from build123d import *

# Parameters (mm, degrees)
SKETCH1_R           = 1.2
BOSS_EXTRUDE1_DEPTH = 1.778
CUT_EXTRUDE1_REACH  = 20.691


with BuildPart() as part:
    # Sketch1 → Boss-Extrude1 (new body)
    with BuildSketch(Plane.XY):
        Polygon((-14.129156365, -0.016893901), (0.010881059, -12.106513676), (14.129156365, 0.016893901), (-0.010881059, 12.106513676), align=None)
        with Locations((0, 8)):
            Circle(SKETCH1_R, mode=Mode.SUBTRACT)
        with Locations((-9.5, 0)):
            Circle(SKETCH1_R, mode=Mode.SUBTRACT)
        with Locations((9.5, 0)):
            Circle(SKETCH1_R, mode=Mode.SUBTRACT)
        with Locations((0, -8)):
            Circle(SKETCH1_R, mode=Mode.SUBTRACT)
    extrude(amount=BOSS_EXTRUDE1_DEPTH)

    # Sketch2 → Cut-Extrude1 (cut, up to next)
    with BuildSketch(Plane.XY.offset(1.778), mode=Mode.PRIVATE) as cut_extrude1_sk1:
        Polygon((-0.003723131, 5.416744003), (-6.321720276, -0.008540092), (0.003723131, -5.416744003), (6.321720276, 0.008540092), align=None)
    cut_extrude1_tool1 = extrude(cut_extrude1_sk1.sketch, amount=-CUT_EXTRUDE1_REACH, mode=Mode.PRIVATE) & part.part
    add(cut_extrude1_tool1.solids().sort_by_distance((0, 0, 1.778))[0], mode=Mode.SUBTRACT)


solid = part.part
CAD build for the part. Positions are in the model's coordinates, mm. A direction names the side the tool comes from. Round coordinates to 2 decimals unless told otherwise and drop trailing zeros. Loops run counter-clockwise (first coordinate to the right, second up) from the corner with the lowest first, then second, coordinate; pieces in that order, holes last.
(1) Two-plate mould, pull along Y, no slides. Class faces 1 (the flat face through (-3, -4, 1.778)), 2 (the flat face through (-6.97, 6.13, 0.88)), 3 (the flat face through (-7.158, -5.977, 0.877)), 4 (the cylindrical face through (-8.355, 0.36, 0.877)): +Y half, -Y half, draft (parallel to the pull), parting line (faces both ways), or undercut.
(2) Cut at C-C (y = -1.75). Give the cut face in (x, z).
(3) Drop flat-ended pins along their axis: pin 1 (1 mm diameter, centred on y = 2.5, z = 1.5, fed in from -X); pin 2 (1.9 mm diameter, centred on x = 0, y = 8, fed in from +Z). Give the stop position or say it passes through.
(4) Cut at A-A (z = 1.2). Give the cut face in (x, y).
(5) Which spindle directions (+Z, -Z, +X, -X, +Y, -Y) get a long thin tool onto all of the face, cutting with end or side? Do faces 5 (the flat face through (7.158, 5.977, 0.877)), 6 (the flat face through (-3.203, -2.675, 0.901)). Say none if no direction does.
(6) Cut at B-B (x = 3). Give the cut face in (y, z).
(7) Wall check: line 1 along Y through (x, z) = (-0.5, 0.3); line 2 along Y through (x, z) = (0.75, 1.35); line 3 along X through (y, z) = (-8.5, 0.8). Give the ranges that are in metal, low to high.
(8) Cut at D-D (y = -6.5). Give the cut face in (x, z).
Findings below:
1. face 1: draft
1. face 2: +Y half
1. face 3: -Y half
1. face 4: undercut
2. outline: (-12.1, 0) - (-4.28, 0) - (-4.28, 1.78) - (-12.1, 1.78) - close; (4.27, 0) - (12.07, 0) - (12.07, 1.78) - (4.27, 1.78) - close
3. pin 1: stops at x = -11.78
3. pin 2: passes through
4. outline: (-14.13, -0.02) - (0.01, -12.11) - (14.13, 0.02) - (-0.01, 12.11) - close; hole circle Ø2.4 at (-9.5, 0); hole (-6.32, -0.01) - (0, -5.42) - (6.32, 0.01) - (0, 5.42) - close; hole circle Ø2.4 at (0, -8); hole circle Ø2.4 at (0, 8); hole circle Ø2.4 at (9.5, 0)
5. face 5: +Z, -Z, +X, +Y
5. face 6: +Z, -Z
6. outline: (-9.54, 0) - (-2.84, 0) - (-2.84, 1.78) - (-9.54, 1.78) - close; (2.85, 0) - (9.53, 0) - (9.53, 1.78) - (2.85, 1.78) - close
7. line 1: y = -11.67 to -9.09, -6.91 to -4.99, 4.99 to 6.91, 9.09 to 11.69
7. line 2: y = -11.47 to -8.94, -7.06 to -4.78, 4.77 to 7.06, 8.94 to 11.46
7. line 3: x = -4.21 to -1.09, 1.09 to 4.21
8. outline: (-6.55, 0) - (6.54, 0) - (6.54, 1.78) - (-6.55, 1.78) - close
